Build history of the part. All positions in model axes, mm. A direction names the side the tool comes from. Coordinates: 2 decimals unless noted, no trailing zeros. Order: outer loops, then holes, each group sorted by start corner. A loop starts at its lowest first (then second) coordinate and runs counter-clockwise, first axis right, second up. Notation, with made-up numbers: (-16.75, 52) - (7.25, 52) arc R24 ccw to (7.25, 83) - close; hole circle Ø10 at (-34.5, -13.5). An arc over 180 degrees is marked (long way). Write each question's results on one line, items separated by ' | '. Start each with the question number.
from build123d import *

# Parameters (mm, degrees)
SKETCH1_W           = 185
SKETCH1_H           = 185
BOSS_EXTRUDE1_DEPTH = 50
CUT_EXTRUDE1_DEPTH  = 190
CUT_EXTRUDE3_START  = -5
CUT_EXTRUDE3_DEPTH  = 175
SKETCH10_W          = 130
SKETCH10_H          = 5
BOSS_EXTRUDE2_DEPTH = 30
SKETCH11_W          = 140
SKETCH11_H          = 5
BOSS_EXTRUDE3_DEPTH = 30


with BuildPart() as part:
    # Sketch1 → Boss-Extrude1 (new body)
    with BuildSketch(Plane.XY):
        with Locations((92.5, -92.5)):
            Rectangle(SKETCH1_W, SKETCH1_H)
    extrude(amount=BOSS_EXTRUDE1_DEPTH)

    # Sketch8 → Cut-Extrude1 (cut)
    with BuildSketch(Plane.XZ.offset(185)):
        Polygon((0, 50), (185, 15), (185, 50), align=None)
    extrude(amount=-CUT_EXTRUDE1_DEPTH, mode=Mode.SUBTRACT)

    # Sketch9 → Cut-Extrude3 (cut)
    with BuildSketch(Plane.XZ.offset(185).offset(CUT_EXTRUDE3_START)):
        Polygon((185, 9.911305302), (5, 43.965359356), (5, 0), (185, 0), align=None)
    extrude(amount=-CUT_EXTRUDE3_DEPTH, mode=Mode.SUBTRACT)

    # Sketch10 → Boss-Extrude2 (add)
    with BuildSketch(Plane.XZ.offset(185)):
        with Locations((65, 17.5)):
            Rectangle(SKETCH10_W, SKETCH10_H)
    extrude(amount=BOSS_EXTRUDE2_DEPTH)

    # Sketch11 → Boss-Extrude3 (add)
    with BuildSketch(Plane(origin=(0, 0, 0), x_dir=(1, 0, 0), z_dir=(0, 1, 0))):
        with Locations((70, -17.5)):
            Rectangle(SKETCH11_W, SKETCH11_H)
    extrude(amount=BOSS_EXTRUDE3_DEPTH)


solid = part.part
Item 1: Flat gauge pins, fed straight in: P1, Ø8, axis at x = 89, y = -39.5, coming from the -Z side; P2, Ø8, axis at x = 165.5, y = -173, coming from the +Z side; P3, Ø2.5, axis at y = -201, z = 18, coming from the +X side. Where does each tip first touch, or does it go through?
Item 2: Probe probe 1 along Y at (x, z) = (63, 17); probe 2 along Y at (x, z) = (46, 26.5); probe 3 along Y at (x, z) = (34, 40). List the from-to ranges inside material, lowest first.
Item 3: Slice it at B-B (x = 39.5). Write the cut outline in (y, z), then the cut area to 3 significant figures.
Item 4: Which spindle directions (+Z, -Z, +X, -X, +Y, -Y) get a long thin tool onto all of the face, cutting with end or side? Do faces 4 (the flat face through (74, -5, 17)), 5 (the flat face through (64, -200, 20)), 6 (the flat face through (69, 15, 15)). Say none if no direction does.
Item 5: Slice it at C-C (y = -18). Write the cut outline in (x, z).
Item 6: Slice it at D-D (z = 39.5). Write the cut outline in (x, y).
Item 7: Slice it at A-A (z = 27.5). Write the cut outline in (x, y).
Item 8: Pull direction Y, two halves, no side cores. Call faces 1 (the flat face through (69, 30, 17)), 2 (the flat face through (5, -94, 22)), 3 (the flat face through (140, 15, 18)): released by +Y, released by -Y, zero draft, split by the parting line, or undercut.
Resolved:
1) P1: z = 27.32 | P2: z = 19.45 | P3: x = 130
2) probe 1: -215 to -180, -5 to 30 | probe 2: -185 to -180, -5 to 0 | probe 3: -185 to 0
3) outline: (-215, 15) - (-185, 15) - (-185, 0) - (-180, 0) - (-180, 37.44) - (-5, 37.44) - (-5, 0) - (0, 0) - (0, 15) - (30, 15) - (30, 20) - (0, 20) - (0, 42.53) - (-185, 42.53) - (-185, 20) - (-215, 20) - close | area: 1,620 mm^2
4) face 4: -Z | face 5: +Z, +X, -X, -Y | face 6: -Z, +X, -X, +Y
5) outline: (0, 0) - (5, 0) - (5, 43.97) - (185, 9.91) - (185, 15) - (0, 50) - close
6) outline: (0, -185) - (55.5, -185) - (55.5, 0) - (0, 0) - close; hole (5, -180) - (28.6, -180) - (28.6, -5) - (5, -5) - close
7) outline: (0, -185) - (118.93, -185) - (118.93, 0) - (0, 0) - close; hole (5, -180) - (92.03, -180) - (92.03, -5) - (5, -5) - close
8) face 1: released by +Y | face 2: undercut | face 3: zero draft
